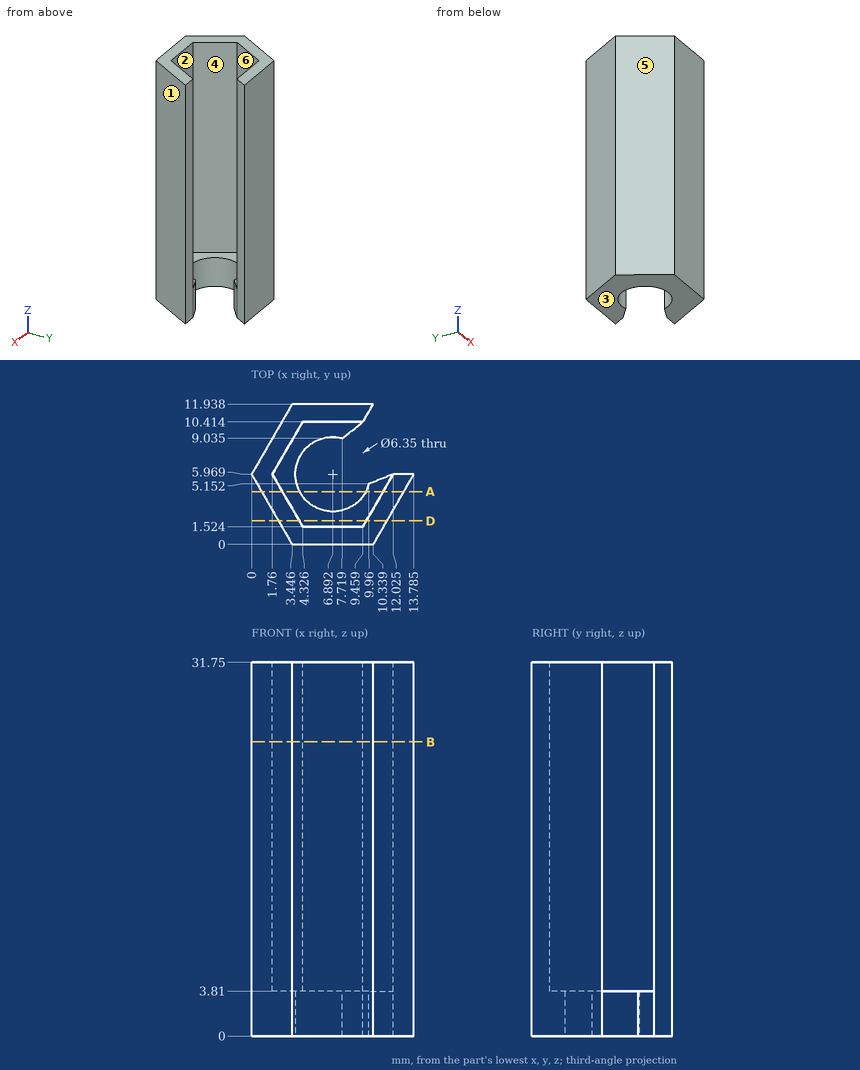
The figure shows three views and two pictorial views of one solid part (mm, origin at its lowest corner). Answer the questions. A direction names the side the tool comes from. Round coordinates to 2 decimals unless told otherwise and drop trailing zeros. Write each loop counter-clockwise with the first axis right and the second up, starting at its lowest first coordinate (ties: lowest second). Pieces come first, ordered by that corner, then holes. Notation, with made-up numbers: (-3.5, 88) - (29.5, 88) arc R25 cw to (29.5, 106) - close; hole circle Ø4 at (2, -31.5). An arc over 180 degrees is marked (long way). Use one line per item in the form item = value. Start each with the question number.
Item 1: A cutting plane is placed at D-D (y = 2). Write down the section's boundary in (x, z).
Item 2: Find the intervals of material crossed by line 1 (Y direction, x = 5, z = 12.5) (1 decimal); line 2 (Z direction, x = 7.75, y = 2.5); line 3 (Y direction, x = 3.75, z = 13.5) (1 decimal), in increasing order. Write a range as [from, to].
Item 3: A tool of negligible diameter and unlimited length cuts with its end or side. For the marked faces 4, 5 and 6, from which of +Z, -Z, +X, -X, +Y, -Y can it reach the whole face along a straight path? Write none if from no direction.
Item 4: Flat-ended cylindrical pins translate along their axes: pin 1 Ø1.4 at (x, z) = (12.5, 20.5) entering from +Y; pin 2 Ø3 at (x, y) = (10.5, 7.5) entering from +Z; pin 3 Ø3 at (y, z) = (6.5, 17) entering from +X (1 decimal); pin 4 Ø5 at (y, z) = (2.5, 6) entering from +X (1 decimal). Find the tip coordinate at first contact, or state that the pin passes through.
Item 5: A cutting plane is placed at B-B (z = 25). Write down the section's boundary in (x, y) (1 decimal).
Item 6: A cutting plane is placed at A-A (y = 4.5). Write down the section's boundary in (x, z), plus the area to 3 significant figures.
Item 7: Determine the mould class of the marked faces 1, 2 and 3 for opening direction X: +X half, -X half, draft (parallel to the pull), parting line (faces both ways), or undercut.
The answers:
q1.outline = (2.29, 0) - (11.49, 0) - (11.49, 31.75) - (9.73, 31.75) - (9.73, 3.81) - (4.05, 3.81) - (4.05, 31.75) - (2.29, 31.75) - close
q2.line_1 = [0, 1.5], [10.4, 11.9]
q2.line_2 = [0, 3.81]
q2.line_3 = [0, 2.5], [9.4, 11.9]
q3.face_4 = +Z
q3.face_5 = +Z, -Z, -X, -Y
q3.face_6 = +Z, +X
q4.pin_1 = 5.97
q4.pin_2 = through
q4.pin_3 = 13.8
q4.pin_4 = 13.2
q5.outline = (0, 6) - (3.4, 0) - (10.3, 0) - (13.8, 6) - (12, 6) - (9.5, 1.5) - (4.3, 1.5) - (1.8, 6) - (4.3, 10.4) - (9.5, 10.4) - (10.3, 11.9) - (3.4, 11.9) - close
q6.outline = (0.85, 0) - (4.08, 0) - (4.08, 3.81) - (2.61, 3.81) - (2.61, 31.75) - (0.85, 31.75) - close; (9.71, 0) - (12.94, 0) - (12.94, 31.75) - (11.18, 31.75) - (11.18, 3.81) - (9.71, 3.81) - close
q6.area = 123 mm^2
q7.face_1 = +X half
q7.face_2 = undercut
q7.face_3 = draft
